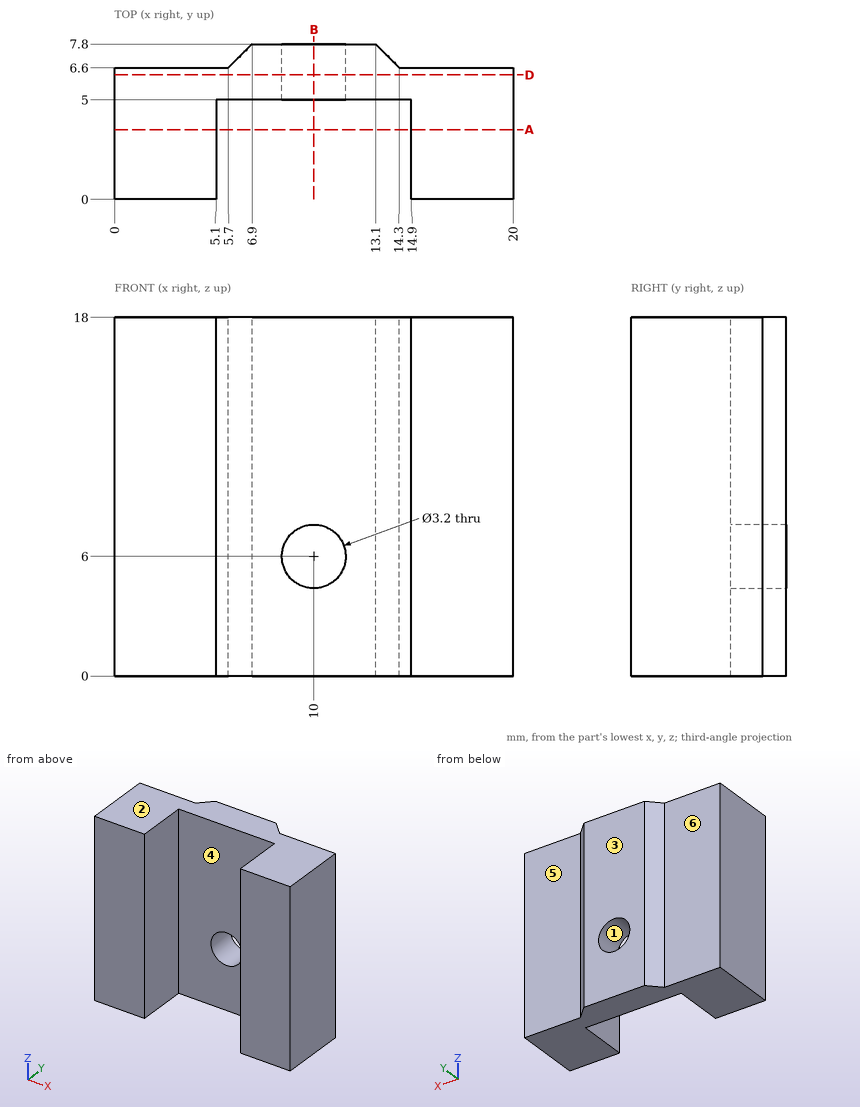
For this review, use the dimensioned drawing (mm, ordinates from the lowest corner) and the shaded views. A direction names the side the tool comes from. Coordinates: 2 decimals unless noted, no trailing zeros. Write each loop counter-clockwise with the first axis right and the second up, starting at its lowest first coordinate (ties: lowest second). Pieces come first, ordered by that corner, then holes. Notation, with made-up numbers: (17.25, 84.5) - (51.25, 84.5) arc R20 ccw to (51.25, 107.5) - close; hole circle Ø3 at (31.5, 22). An arc over 180 degrees is marked (long way). One line per item, written item: value.
1) Add section A-A (y = 3.5). State the section outline as (x, z) points, plus the area to 3 significant figures.
Answer sheet:
outline: (0, 0) - (5.1, 0) - (5.1, 18) - (0, 18) - close; (14.9, 0) - (20, 0) - (20, 18) - (14.9, 18) - close
area: 184 mm2
2) Add section B-B (x = 10). State the section outline as (y, z) points, plus the area to 3 significant figures.
Answer sheet:
outline: (5, 0) - (7.8, 0) - (7.8, 4.4) - (5, 4.4) - close; (5, 7.6) - (7.8, 7.6) - (7.8, 18) - (5, 18) - close
area: 41.4 mm2
3) To check wall thickness, follow probe 1 along X at (y, z) = (3.5, 14); probe 2 along X at (y, z) = (5.95, 6); probe 3 along Y at (x, z) = (4.25, 7). State the ranges of each line that lie inside material, in increasing order.
Answer sheet:
probe 1: x = 0 to 5.1, 14.9 to 20
probe 2: x = 0 to 8.4, 11.6 to 20
probe 3: y = 0 to 6.6
4) Insertion check: pin 1 (5 mm diameter, centred on x = 9, z = 6, fed in from -Y); pin 2 (1.7 mm diameter, centred on x = 16, z = 9.5, fed in from +Y); pin 3 (1.9 mm diameter, centred on x = 10, z = 6, fed in from -Y). Each pin has a flat end and moves straight along its axis. Give the tip position at first contact, or say it passes through.
Answer sheet:
pin 1: stops at y = 5
pin 2: stops at y = 6.6
pin 3: passes through
5) Add section D-D (y = 6.25). State the section outline as (x, z) points.
Answer sheet:
outline: (0, 0) - (20, 0) - (20, 18) - (0, 18) - close; hole circle Ø3.2 at (10, 6)
6) Mouldability with a two-part tool opening along Z and no side actions: class the marked faces 1, 2 and 3 as +Z half, -Z half, draft (parallel to the pull), parting line (faces both ways), or undercut.
Answer sheet:
face 1: undercut
face 2: +Z half
face 3: draft
7) For the marked faces 4, 5 and 6, list the 3-axis set-ups (+Z, -Z, +X, -X, +Y, -Y) from which the entire face can be reached by the end or side of a thin tool; tool diameter is ignored.
Answer sheet:
face 4: +Z, -Z, -Y
face 5: +Z, -Z, +X, +Y
face 6: +Z, -Z, -X, +Y
